Source: CAD feature listing. Evaluate the final solid. Frame: model axes, mm. A direction names the side the tool comes from. Coordinates: 2 decimals unless noted, no trailing zeros. Order: outer loops, then holes, each group sorted by start corner. A loop starts at its lowest first (then second) coordinate and runs counter-clockwise, first axis right, second up.
Item 1: Mould query, pull axis Z, two halves, no side actions, for faces 4 (the cylindrical face through (0, 1, -20)), 5 (the flat face through (0, 1, 20)), 6 (the flat face through (13.5, 2, 9)), 7 (the flat face through (0, 3, 0)). Classes: released by +Z, released by -Z, zero draft, split by the parting line, or undercut.
Item 2: Ray query, line 1 (Z direction, x = -15, y = 1.4); line 2 (Z direction, x = -16, y = 2.4); line 3 (X direction, y = 2.65, z = 4.5). Return the intervals inside material, ascending.
Item 3: Reachability of faces 1 (the flat face through (-16, 2, 2.5)), 2 (the flat face through (16, 2, 2.5)), 3 (the flat face through (0, 0, 0)) from +Z, -Z, +X, -X, +Y, -Y: full face, straight path, thin tool, end or side. Return the list, or none.
Item 4: Section C-C on x = 7.5. Return the cut outline in (y, z).
Item 5: Section B-B on z = -12. Return the cut outline in (x, y), then the cut area to 3 significant figures.
Item 6: Contact query for flat-ended pins moving along their axis: P1, Ø0.9, axis at y = 1.5, z = 10.5, coming from the -X side; P2, Ø1, axis at y = 2, z = -15.5, coming from the -X side; P3, Ø0.9, axis at x = -16.5, y = 2, coming from the -Z side. Output: stop coordinate, or through.
Item 7: Section A-A on y = 1.35. Return the cut outline in (x, z), then the cut area to 3 significant figures.
from build123d import *

# Parameters (mm, degrees)
BOSS_EXTRUDE1_DEPTH = 3
SKETCH2_W           = 5
SKETCH2_H           = 13
CUT_EXTRUDE2_DEPTH  = 10


with BuildPart() as part:
    # Sketch1 → Boss-Extrude1 (new body)
    with BuildSketch(Plane(origin=(0, 0, 0), x_dir=(1, 0, 0), z_dir=(0, 1, 0))):
        with BuildLine():
            ThreePointArc((18.5, 7.599342077), (0, 20), (-18.5, 7.599342077))
            Line((-18.5, 7.599342077), (-18.5, -20))
            Line((-18.5, -20), (18.5, -20))
            Line((18.5, -20), (18.5, 7.599342077))
        make_face()
    extrude(amount=BOSS_EXTRUDE1_DEPTH)

    # Sketch2 → Cut-Extrude2 (cut)
    with BuildSketch(Plane(origin=(0, 3, 0), x_dir=(1, 0, 0), z_dir=(0, 1, 0))):
        with Locations((-16, -9)):
            Rectangle(SKETCH2_W, SKETCH2_H)
        with Locations((16, -9)):
            Rectangle(SKETCH2_W, SKETCH2_H)
    extrude(amount=-CUT_EXTRUDE2_DEPTH, mode=Mode.SUBTRACT)


solid = part.part
Answer list:
1. face 4: released by -Z
1. face 5: released by +Z
1. face 6: undercut
1. face 7: zero draft
2. line 1: z = -13.23 to 2.5, 15.5 to 20
2. line 2: z = -12 to 2.5, 15.5 to 20
2. line 3: x = -13.5 to 13.5
3. face 1: -X, +Y, -Y
3. face 2: +X, +Y, -Y
3. face 3: +Z, -Z, +X, -X, -Y
4. outline: (0, -18.54) - (3, -18.54) - (3, 20) - (0, 20) - close
5. outline: (-16, 0) - (16, 0) - (16, 3) - (-16, 3) - close
5. area: 96.0 mm2
6. P1: stops at x = -13.5
6. P2: stops at x = -13.23
6. P3: stops at z = -11.93
7. outline: (-18.5, -7.6) arc R20 ccw to (18.5, -7.6) - (18.5, 2.5) - (13.5, 2.5) - (13.5, 15.5) - (18.5, 15.5) - (18.5, 20) - (-18.5, 20) - (-18.5, 15.5) - (-13.5, 15.5) - (-13.5, 2.5) - (-18.5, 2.5) - close
7. area: 1,220 mm2
